Work out the finished part from the listing and answer in its coordinate system (mm). Face numbers are marked on the shaded views. A direction names the side the tool comes from. Coordinates: 2 decimals unless noted, no trailing zeros. Loops run counter-clockwise (first coordinate to the right, second up) from the corner with the lowest first, then second, coordinate; pieces in that order, holes last. Notation, with made-up numbers: (10.5, 66.25) -> (45.5, 66.25) arc R22 ccw to (45.5, 88.25) -> close; hole circle Ø1 at (-17, -4.75). An arc over 180 degrees is marked (long way). One line per question, with ' | ' between items.
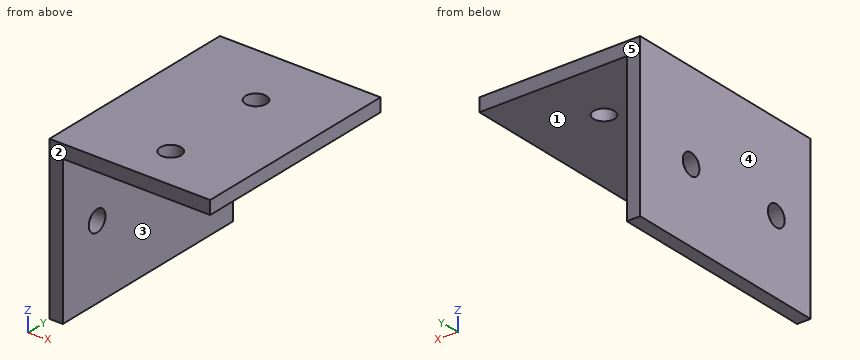
```python
from build123d import *

# Parameters (mm, degrees)
EXTRUDE_THIN1_DEPTH = 25.4
SKETCH2_R           = 2.4892
CUT_EXTRUDE1_DEPTH  = 4.175


with BuildPart() as part:
    # Sketch1 → Extrude-Thin1 (new body, symmetric)
    with BuildSketch(Plane(origin=(0, 0, 0), x_dir=(1, 0, 0), z_dir=(0, 1, 0))):
        Polygon((0, 38.1), (0, 0), (38.1, 0), (38.1, 3.175), (3.175, 3.175), (3.175, 38.1), align=None)
    extrude(amount=EXTRUDE_THIN1_DEPTH, both=True)

    # Sketch2 → Cut-Extrude1 (cut, through all)
    with BuildSketch(Plane(origin=(0, 0, -3.175), x_dir=(-1, 0, 0), z_dir=(0, 0, -1))):
        with Locations((-20.6375, 10.2108)):
            Circle(SKETCH2_R)
        with Locations((-20.6375, -15.1892)):
            Circle(SKETCH2_R)
    cut_extrude1 = extrude(amount=-CUT_EXTRUDE1_DEPTH, mode=Mode.SUBTRACT)

    # Mirror1: Cut-Extrude1 across plane
    add(cut_extrude1.mirror(Plane(origin=(0, 0, 0), x_dir=(-0.707106781, 0, 0.707106781), z_dir=(-0.707106781, 0, -0.707106781))), mode=Mode.SUBTRACT)


solid = part.part
```
1) Find section C-C (y = -6). Write down the section's boundary in (x, z) (3 decimals).
Check values:
outline: (0, -38.1) -> (3.175, -38.1) -> (3.175, -3.175) -> (38.1, -3.175) -> (38.1, 0) -> (0, 0) -> close
2) Find section B-B (z = -20). Write down the section's boundary in (x, y) (3 decimals), plus the area to 3 significant figures.
Check values:
outline: (0, -25.4) -> (3.175, -25.4) -> (3.175, -17.595) -> (0, -17.595) -> close; (0, -12.783) -> (3.175, -12.783) -> (3.175, 7.805) -> (0, 7.805) -> close; (0, 12.617) -> (3.175, 12.617) -> (3.175, 25.4) -> (0, 25.4) -> close | area: 131 mm^2
3) Find the intervals of material crossed by line 1 along X through (y, z) = (-1.5, -5) (3 decimals); line 2 along Z through (x, y) = (17, 18) (3 decimals), in increasing order.
Check values:
line 1: x = 0 to 3.175 | line 2: z = -3.175 to 0
4) Find section A-A (y = -13.5). Write down the section's boundary in (x, z) (3 decimals), plus the area to 3 significant figures.
Check values:
outline: (0, -38.1) -> (3.175, -38.1) -> (3.175, -22.466) -> (0, -22.466) -> close; (0, -18.809) -> (3.175, -18.809) -> (3.175, -3.175) -> (18.809, -3.175) -> (18.809, 0) -> (0, 0) -> close; (22.466, -3.175) -> (38.1, -3.175) -> (38.1, 0) -> (22.466, 0) -> close | area: 209 mm^2
5) Flat-ended cylindrical pins translate along their axes: pin 1 (6.5 mm diameter, centred on x = 20.64, y = 10.21, fed in from -Z) (3 decimals); pin 2 (12 mm diameter, centred on y = -19, z = -18.5, fed in from +X) (3 decimals). Find the tip coordinate at first contact, or state that the pin passes through.
Check values:
pin 1: stops at z = -3.175 | pin 2: stops at x = 3.175
6) Find section D-D (x = 4.5). Write down the section's boundary in (y, z) (3 decimals).
Check values:
outline: (-25.4, -3.175) -> (25.4, -3.175) -> (25.4, 0) -> (-25.4, 0) -> close
7) The mould has two halves that part along X. Classify the marked faces 3, 4 and 5: released by +X, released by -X, zero draft, split by the parting line, or undercut.
Check values:
face 3: released by +X | face 4: released by -X | face 5: zero draft
8) For the marked faces 1 and 2, determine the directions among +Z, -Z, +X, -X, +Y, -Y from which every point of the face is accessible in a straight line to the end or side of a thin tool.
Check values:
face 1: -Z, +X, +Y, -Y | face 2: +Z, -Z, +X, -X, -Y
